Design review of the part built by this model. Coordinates are the model's own, in mm. Face numbers are marked on the shaded views. A direction names the side the tool comes from. Coordinates: 2 decimals unless noted, no trailing zeros. Loops run counter-clockwise (first coordinate to the right, second up) from the corner with the lowest first, then second, coordinate; pieces in that order, holes last. Notation, with made-up numbers: M -8,35.5 L -2,35.5 A14 ccw -2,59.5 Z; hole C 21.25,72 d8. An arc over 180 degrees is marked long. Put each result on its own line as item: value. Start each with the question number.
(1) Take a section at A-A, the plane z = 48. Give the boundary of the cut face in (x, y).
(2) Take a section at D-D, the plane x = 82.5. Give the boundary of the cut face in (y, z), then the cut area to 3 significant figures.
(3) Take a section at C-C, the plane z = 13. Give the boundary of the cut face in (x, y).
(4) The part is to be moulded in two halves that separate along X. For the marked faces 1, 2 and 3, say which applies: +X half, -X half, draft (parallel to the pull), parting line (faces both ways), or undercut.
(5) Clearance check with flat-ended pins moving along their axes: pin 1 (10 mm diameter, centred on y = 30, z = 38, fed in from +X); pin 2 (12 mm diameter, centred on y = 29, z = 24.5, fed in from -X); pin 3 (8 mm diameter, centred on y = 9.5, z = 15.5, fed in from +X); pin 4 (4 mm diameter, centred on x = 27.5, z = 38, fed in from +Y). State where each tip first meets the part, or that it passes through.
(6) For probe 1 along Y at (x, z) = (41, 38); probe 2 along Y at (x, z) = (75, 5.5); probe 3 along X at (y, z) = (19, 32), list the stretches that pass through material, from the lowest coordinate up. Write a range as [from, to].
(7) For the marked faces 4, 5 and 6, list the 3-axis set-ups (+Z, -Z, +X, -X, +Y, -Y) from which the entire face can be reached by the end or side of a thin tool; tool diameter is ignored.
(8) Take a section at B-B, the plane y = 25. Give the boundary of the cut face in (x, z).
```python
from build123d import *

# Parameters (mm, degrees)
F1_DEPTH  = 50
F3_DEPTH  = 81.2
F4_DEPTH  = 25
F5_W      = 49.6666632582
F5_H      = 56
F6_DEPTH  = 41.9
F7_W      = 49.6666632582
F7_H      = 17.3173451722
F8_DEPTH  = 28.3
F10_DEPTH = 17.2


with BuildPart() as f1:
    # F0 (on Top) → F1 (new body)
    with BuildSketch(Plane.XY):
        Polygon((102.878117487, 58), (0, 58), (0, 0), (58, 0), (58, 16), (16, 16), (16, 42), (88, 42), (88, 16), (102.878117487, 16), align=None)
        Polygon((16, 16), (58, 16), (88, 16), (88, 42), (16, 42), align=None)
    extrude(amount=F1_DEPTH)

    # F2 (on face) → F3 (cut)
    with BuildSketch(Plane.XZ):
        Polygon((58, 50), (0, 50), (58, 25.4237288136), align=None)
        Polygon((58, 50), (58, 25.4237288136), (118, 0), (102.9013991356, 50), align=None)
    extrude(amount=-F3_DEPTH, mode=Mode.SUBTRACT)

    # F2 (on face) → F4 (cut)
    with BuildSketch(Plane.XZ):
        Polygon((58, 50), (58, 25.4237288136), (118, 0), (102.9013991356, 50), align=None)
    extrude(amount=-F4_DEPTH, mode=Mode.SUBTRACT)

    # F5 (on face) → F6 (join)
    with BuildSketch(Plane(origin=(0, 58, 0), x_dir=(-1, 0, 0), z_dir=(0, 1, 0))):
        with Locations((-36.3266665494, 28)):
            Rectangle(F5_W, F5_H)
    extrude(amount=-F6_DEPTH)

    # F7 (on face) → F8 (cut)
    with BuildSketch(Plane.XY.offset(56)):
        with Locations((36.3266665494, 49.3413274139)):
            Rectangle(F7_W, F7_H)
    extrude(amount=-F8_DEPTH, mode=Mode.SUBTRACT)

    # F9 (on face) → F10 (join)
    with BuildSketch(Plane(origin=(0, 40.6826548278, 0), x_dir=(-1, 0, 0), z_dir=(0, 1, 0))):
        Polygon((-11.4933349202, 45.1299428304), (-61.1599981785, 27.7), (-11.4933349202, 27.7), align=None)
    extrude(amount=F10_DEPTH)


solid = f1.part
```
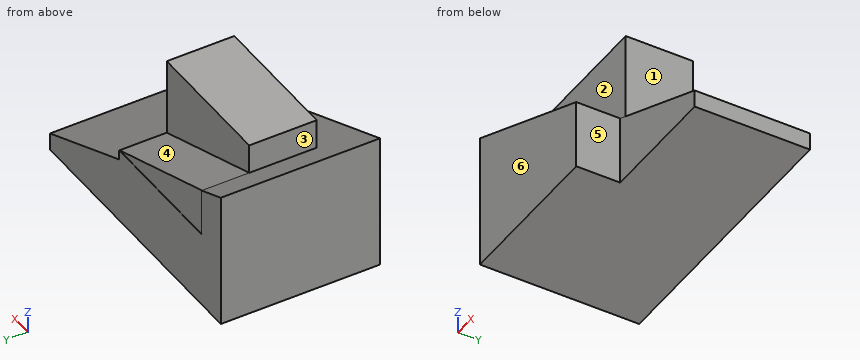
Computed values:
1. outline: M 0,0 L 4.72,0 L 4.72,58 L 0,58 Z; M 11.49,16.1 L 61.16,16.1 L 61.16,40.68 L 11.49,40.68 Z
2. outline: M 16,0 L 58,0 L 58,15.04 L 16,15.04 Z
2. area: 632 mm^2
3. outline: M 0,0 L 58,0 L 58,16 L 87.32,16 L 87.32,58 L 0,58 Z
4. face 1: +X half
4. face 2: draft
4. face 3: undercut
5. pin 1: stops at x = 61.16
5. pin 2: stops at x = 0
5. pin 3: stops at x = 58
5. pin 4: stops at y = 57.88
6. probe 1: y = [16.1, 40.68]
6. probe 2: y = [16, 58]
6. probe 3: x = [0, 61.16]
7. face 4: +Z, +X, +Y
7. face 5: +Z, -Z, +X, -Y
7. face 6: +Z, -Z, +X, -X, -Y
8. outline: M 0,0 L 102.88,0 L 102.88,6.41 L 61.16,24.08 L 61.16,56 L 11.49,56 L 11.49,45.13 L 0,50 Z
